Design review of the part built by this model. Coordinates are the model's own, in mm. A direction names the side the tool comes from. Coordinates: 2 decimals unless noted, no trailing zeros. Loops run counter-clockwise (first coordinate to the right, second up) from the corner with the lowest first, then second, coordinate; pieces in that order, holes last. Notation, with made-up numbers: (78, -36) - (84, -36) arc R22 cw to (84, 1) - close; hole circle Ø2 at (35.5, 87.25). An arc over 180 degrees is marked (long way). Answer in a Markdown table with one row per item. Add a question column.
(1) To check wall thickness, follow L1, parallel to X at y = 3.75, z = 41.5 (3 decimals); L2, parallel to X at y = 4.25, z = 18; L3, parallel to Y at x = 0, z = 49. State the ranges of each line that lie inside material, in increasing order. Write a range as [from, to].
(2) The part is to be moulded in two halves that separate along X. For faces 5 (the face through (14, -6, 3.091)), 6 (the face through (-25.4, 0, 25)), 7 (the face through (5, 6.35, 25)), say which applies: released by +X, released by -X, zero draft, split by the parting line, or undercut.
(3) Clearance check with a flat-ended pin moving along its axis: pin 1 (4 mm diameter, centred on x = 8, z = 16.5, fed in from -Y). State where the tip first meets the part, or that it passes through.
(4) We need section C-C, the plane y = 0. Write out the cut boundary in (x, z) (3 decimals).
(5) For faces 1 (the face through (-0.4, 4.3, 50.8)), 2 (the face through (-3, 3, 45.72)), 3 (the face through (0, 5, 39.37)), 4 (the face through (-13, -4.762, 26)), list the 3-axis set-ups (+Z, -Z, +X, -X, +Y, -Y) from which the entire face can be reached by the end or side of a thin tool; tool diameter is ignored.
(6) We need section A-A, the plane x = 0. Write out the cut boundary in (y, z), plus the area to 3 significant figures.
from build123d import *

# Parameters (mm, degrees)
F0_W      = 50.8
F0_H      = 12.7
F1_DEPTH  = 50.8
F3_START  = -5.08
F2_W      = 6.35
F2_H      = 7.62
F3_DEPTH  = 39.37
F4_R      = 3.91795
F5_DEPTH  = 6.35
F6_W      = 4.7625
F6_H      = 27.94
F7_DEPTH  = 12.701
F8_W      = 19.05
F8_H      = 45.72
F9_DEPTH  = 1.5875
F10_W     = 19.05
F10_H     = 45.72
F11_DEPTH = 1.5875


with BuildPart() as f1:
    # F0 (on Top) → F1 (new body)
    with BuildSketch(Plane.XY):
        Rectangle(F0_W, F0_H)
    extrude(amount=F1_DEPTH)

    # F2 (on face) → F3 (cut)
    with BuildSketch(Plane.XY.offset(50.8).offset(F3_START)):
        Rectangle(F2_W, F2_H)
    extrude(amount=-F3_DEPTH, mode=Mode.SUBTRACT)

    # F4 (on face) → F5 (cut)
    with BuildSketch(Plane.XY.offset(50.8)):
        Circle(F4_R)
    extrude(amount=-F5_DEPTH, mode=Mode.SUBTRACT)

    # F6 (on face) → F7 (cut, through all)
    with BuildSketch(Plane.XZ.offset(6.35)):
        with Locations((0, 25.4)):
            Rectangle(F6_W, F6_H)
    extrude(amount=-F7_DEPTH, mode=Mode.SUBTRACT)

    # F8 (on face) → F9 (cut)
    with BuildSketch(Plane.XZ.offset(6.35)):
        with Locations((-13.3303813094, 25.6625675702)):
            Rectangle(F8_W, F8_H)
    extrude(amount=-F9_DEPTH, mode=Mode.SUBTRACT)

    # F10 (on face) → F11 (cut)
    with BuildSketch(Plane.XZ.offset(6.35)):
        with Locations((14.600383172, 25.9514273362)):
            Rectangle(F10_W, F10_H)
    extrude(amount=-F11_DEPTH, mode=Mode.SUBTRACT)


solid = f1.part
Responses:
| question | item | result |
|---|---|---|
| 1 | L1 | x = [-25.4, -3.175], [3.175, 25.4] |
| 1 | L2 | x = [-25.4, -2.38], [2.38, 25.4] |
| 1 | L3 | y = [-6.35, -3.92], [3.92, 6.35] |
| 2 | face 5 | undercut |
| 2 | face 6 | released by -X |
| 2 | face 7 | zero draft |
| 3 | pin 1 | stops at y = -4.76 |
| 4 | outline | (-25.4, 0) - (25.4, 0) - (25.4, 50.8) - (3.918, 50.8) - (3.918, 44.45) - (3.175, 44.45) - (3.175, 6.35) - (-3.175, 6.35) - (-3.175, 44.45) - (-3.918, 44.45) - (-3.918, 50.8) - (-25.4, 50.8) - close |
| 5 | face 1 | +Z, +X, -X, +Y, -Y |
| 5 | face 2 | none |
| 5 | face 3 | +Y, -Y |
| 5 | face 4 | -Y |
| 6 | outline | (-6.35, 0) - (6.35, 0) - (6.35, 11.43) - (3.81, 11.43) - (3.81, 6.35) - (-3.81, 6.35) - (-3.81, 11.43) - (-6.35, 11.43) - close; (-6.35, 39.37) - (-3.81, 39.37) - (-3.81, 44.45) - (-3.92, 44.45) - (-3.92, 50.8) - (-6.35, 50.8) - close; (3.81, 39.37) - (6.35, 39.37) - (6.35, 50.8) - (3.92, 50.8) - (3.92, 44.45) - (3.81, 44.45) - close |
| 6 | area | 163 mm2 |
